from build123d import *

# Parameters (mm, degrees)
SKETCH1_W               = 129
SKETCH1_H               = 20
BOSS_EXTRUDE1_DEPTH     = 8
SKETCH2_W               = 13
SKETCH2_H               = 15
SKETCH2_W_2             = 12
SKETCH2_H_2             = 13
CUT_EXTRUDE4_DEPTH      = 3.6
SKETCH2_5_R             = 2.25
CUT_EXTRUDE7_DEPTH      = 131.786084887
CUT_EXTRUDE8_DEPTH      = 131.615313038
CUT_EXTRUDE8_DEPTH_BACK = 131.615313038
SKETCH3_W               = 13
SKETCH3_H               = 3
CUT_EXTRUDE9_DEPTH      = 5
CHAMFER1_SIZE           = 1
SKETCH5_W               = 42
SKETCH5_H               = 20
SKETCH5_W_2             = 2
SKETCH5_H_2             = 8
CUT_EXTRUDE10_DEPTH     = 2.5
CHAMFER2_DEPTH          = 20
SKETCH6_W               = 5
SKETCH6_H               = 4.5
SKETCH6_W_2             = 8
SKETCH6_H_2             = 3.5
CUT_EXTRUDE11_DEPTH     = 4
SKETCH7_W               = 20
SKETCH7_H               = 4
SKETCH7_W_2             = 10
SKETCH7_W_3             = 5
SKETCH7_H_2             = 5
BOSS_EXTRUDE2_DEPTH     = 2.5
CHAMFER3_SIZE           = 1
FILLET1_R               = 2
CHAMFER4_SIZE           = 1


with BuildPart() as part:
    # Sketch1 → Boss-Extrude1 (new body)
    with BuildSketch(Plane.XY):
        with Locations((64.5, 10)):
            Rectangle(SKETCH1_W, SKETCH1_H)
    extrude(amount=BOSS_EXTRUDE1_DEPTH)

    # Sketch2 → Cut-Extrude4 (cut)
    with BuildSketch(Plane.XY.offset(8)):
        with Locations((12.5, 8.5)):
            Rectangle(SKETCH2_W, SKETCH2_H)
        with Locations((55, 9.5)):
            Rectangle(SKETCH2_W_2, SKETCH2_H_2)
        with Locations((34, 9.5)):
            Rectangle(SKETCH2_W_2, SKETCH2_H_2)
        with Locations((76, 9.5)):
            Rectangle(SKETCH2_W_2, SKETCH2_H_2)
        with Locations((97, 9.5)):
            Rectangle(SKETCH2_W_2, SKETCH2_H_2)
        with BuildLine():
            Line((112, 16), (112, 3))
            Line((112, 3), (123.75, 3))
            ThreePointArc((123.75, 3), (123.813393039, 3.530330086), (124, 4.030776406))
            Line((124, 4.030776406), (124, 15.969223594))
            ThreePointArc((124, 15.969223594), (123.992158813, 15.984581975), (123.984435563, 16))
            Line((123.984435563, 16), (112, 16))
        make_face()
    extrude(amount=-CUT_EXTRUDE4_DEPTH, mode=Mode.SUBTRACT)

    # Sketch2<5> → Cut-Extrude7 (cut, through all)
    with BuildSketch(Plane.XY.offset(8)):
        with Locations((126, 3)):
            Circle(SKETCH2_5_R)
        with Locations((126, 17)):
            Circle(SKETCH2_5_R)
        with Locations((3, 17)):
            Circle(SKETCH2_5_R)
        with Locations((3, 3)):
            Circle(SKETCH2_5_R)
    extrude(amount=-CUT_EXTRUDE7_DEPTH, mode=Mode.SUBTRACT)

    # Sketch3 → Cut-Extrude8 (cut, two sides: drawn at the far end of the back side and taken through both)
    with BuildSketch(Plane.XY.offset(4.4).offset(-CUT_EXTRUDE8_DEPTH_BACK)):
        with Locations((12.5, 1.5)):
            Rectangle(SKETCH3_W, SKETCH3_H)
    extrude(amount=CUT_EXTRUDE8_DEPTH + CUT_EXTRUDE8_DEPTH_BACK, mode=Mode.SUBTRACT)

    # Sketch4 → Cut-Extrude9 (cut)
    with BuildSketch(Plane(origin=(0, 0, 0), x_dir=(-1, 0, 0), z_dir=(0, 0, -1))):
        with BuildLine():
            Line((-28.5, 4.596136616), (-28.5, 15.403863384))
            ThreePointArc((-28.5, 15.403863384), (-24.5, 19.403863384), (-20.5, 15.403863384))
            Line((-20.5, 15.403863384), (-20.5, 4.596136616))
            ThreePointArc((-20.5, 4.596136616), (-24.5, 0.596136616), (-28.5, 4.596136616))
        make_face()
    extrude(amount=-CUT_EXTRUDE9_DEPTH, mode=Mode.SUBTRACT)

    # Chamfer1
    # the kernel refuses this chamfer: 1 mm, written as the material it takes off along each edge
    with BuildSketch(Plane(origin=(24.5, 4.596136616, 0), x_dir=(-1, 0, 0), z_dir=(0, 1, 0))) as chamfer1_piece_1:
        Polygon((4 + CHAMFER1_SIZE, 0), (4, CHAMFER1_SIZE), (4, 0), align=None)
    revolve(axis=Axis((24.5, 4.596136616, 0), (0, 0, 1)), revolution_arc=180, mode=Mode.SUBTRACT)
    with BuildSketch(Plane(origin=(20.5, 15.403863384, 0), x_dir=(-1, 0, 0), z_dir=(0, -1, 0)), Plane(origin=(28.5, 4.596136616, 0), x_dir=(1, 0, 0), z_dir=(0, 1, 0))) as chamfer1_piece_2:
        Polygon((CHAMFER1_SIZE, 0), (0, -CHAMFER1_SIZE), (0, 0), align=None)
    extrude(amount=10.807726767, mode=Mode.SUBTRACT)
    with BuildSketch(Plane(origin=(24.5, 15.403863384, 0), x_dir=(1, 0, 0), z_dir=(0, -1, 0))) as chamfer1_piece_3:
        Polygon((4 + CHAMFER1_SIZE, 0), (4, CHAMFER1_SIZE), (4, 0), align=None)
    revolve(axis=Axis((24.5, 15.403863384, 0), (0, 0, 1)), revolution_arc=180, mode=Mode.SUBTRACT)

    # Sketch5 → Cut-Extrude10 (cut)
    with BuildSketch(Plane(origin=(0, 0, 0), x_dir=(-1, 0, 0), z_dir=(0, 0, -1))):
        with Locations((-49.5, 10)):
            Rectangle(SKETCH5_W, SKETCH5_H)
        with Locations((-1, 10)):
            Rectangle(SKETCH5_W_2, SKETCH5_H_2)
    extrude(amount=-CUT_EXTRUDE10_DEPTH, mode=Mode.SUBTRACT)

    # Chamfer2: read off the stored shape, not the designer's step
    # Chamfer2 outline → Chamfer2 (add)
    with BuildSketch(Plane(origin=(0, 0, 0), x_dir=(1, 0, 0), z_dir=(0, 1, 0))):
        Polygon((28.5, -1), (28.5, -2.5), (30, -2.5), align=None)
    extrude(amount=CHAMFER2_DEPTH)

    # Sketch6 → Cut-Extrude11 (cut)
    with BuildSketch(Plane(origin=(0, 0, 0), x_dir=(-1, 0, 0), z_dir=(0, 0, -1))):
        with Locations((-88.5, 4.75)):
            Rectangle(SKETCH6_W, SKETCH6_H)
        Polygon((-113, 2.5), (-108, 2.5), (-108, 12.5), (-113, 12.5), (-113, 10), (-113, 6), align=None)
        with Locations((-117, 4.25)):
            Rectangle(SKETCH6_W_2, SKETCH6_H_2)
        Polygon((-121, 6), (-113, 6), (-113, 10), (-129, 10), (-129, 6), align=None)
        Polygon((-113, 10), (-113, 12.5), (-113, 14), (-129, 14), (-129, 10), align=None)
    extrude(amount=-CUT_EXTRUDE11_DEPTH, mode=Mode.SUBTRACT)

    # Sketch7 → Boss-Extrude2 (add)
    with BuildSketch(Plane(origin=(0, 0, 2.5), x_dir=(-1, 0, 0), z_dir=(0, 0, -1))):
        with Locations((-60.5, 2)):
            Rectangle(SKETCH7_W, SKETCH7_H)
        with Locations((-65.5, 18)):
            Rectangle(SKETCH7_W_2, SKETCH7_H)
        with Locations((-43.5, 8.5)):
            Rectangle(SKETCH7_W_3, SKETCH7_H_2)
    extrude(amount=BOSS_EXTRUDE2_DEPTH)

    # Chamfer3
    chamfer3_edges = [part.edges().sort_by_distance(p)[0] for p in [
        (0, 14, 1.25),
        (0, 6, 1.25),
    ]]
    chamfer(chamfer3_edges, length=CHAMFER3_SIZE)

    # Fillet1
    fillet1_edges = [part.edges().sort_by_distance(p)[0] for p in [
        (112, 3, 6.2),
        (112, 16, 6.2),
        (70, 16, 6.2),
        (82, 16, 6.2),
        (82, 3, 6.2),
        (70, 3, 6.2),
        (40, 16, 6.2),
        (40, 3, 6.2),
        (61, 16, 6.2),
        (61, 3, 6.2),
        (49, 3, 6.2),
        (49, 16, 6.2),
        (103, 16, 6.2),
        (103, 3, 6.2),
        (91, 3, 6.2),
        (91, 16, 6.2),
    ]]
    fillet(fillet1_edges, radius=FILLET1_R)

    # Chamfer4
    chamfer4_edges = [part.edges().sort_by_distance(p)[0] for p in [
        (0, 20, 4),
        (129, 20, 4),
        (129, 0, 4),
        (0, 0, 4),
    ]]
    chamfer(chamfer4_edges, length=CHAMFER4_SIZE)


solid = part.part
Input: part model. Units: mm. Frame: model coordinates. A direction names the side the tool comes from. Coordinates: 2 decimals unless noted, no trailing zeros. Order: outer loops, then holes, each group sorted by start corner. A loop starts at its lowest first (then second) coordinate and runs counter-clockwise, first axis right, second up. Notation, with made-up numbers: M 82.5,52.5 L 134.5,52.5 A24 ccw 134.5,75.5 Z; hole C 24,-33 d6. An arc over 180 degrees is marked long. Answer as CSV lines item,"result".
1. Material intervals for line 1 (Y direction, x = 3, z = 5.5); line 2 (Y direction, x = 126, z = 3.25); line 3 (X direction, y = 6.5, z = 1.25), sorted ascending. Write a range as from..to.
Reported:
line 1,"0..0.75, 5.25..14.75, 19.25..20"
line 2,"0..0.75, 5.25..6, 14..14.75, 19.25..20"
line 3,"2..20.5, 28.5..28.75, 41..46, 70.5..86, 91..108"
2. Section B-B (x = 74.5). Return the cut outline in (y, z), then the cut area to 3 significant figures.
Reported:
outline,"M 0,0 L 20,0 L 20,8 L 16,8 L 16,4.4 L 3,4.4 L 3,8 L 0,8 Z"
area,"113 mm2"
3. Section D-D (x = 24.5). Return the cut outline in (y, z).
Reported:
outline,"M 0,0.4 L 0.6,1 L 0.6,5 L 19.4,5 L 19.4,1 L 20,0.4 L 20,8 L 0,8 Z"
4. Access query for faces 1 (the flat face through (76, 3, 6)), 2 (the flat face through (12, 10, 4.4)), 3 (the flat face through (46, 8, 1)), 4 (the flat face through (1, 10, 2.5)). Directions: +Z, -Z, +X, -X, +Y, -Y. A direction counts if a zero-diameter tool reaches every point of the face in a straight line with its end or side. Return the directions, or none.
Reported:
face 1,"+Z"
face 2,"+Z, -Y"
face 3,"-Z, +Y, -Y"
face 4,"-Z, -X"
5. Section A-A (x = 126). Return the cut outline in (y, z).
Reported:
outline,"M 0,0 L 0.75,0 L 0.75,8 L 0,8 Z; M 5.25,0 L 6,0 L 6,4 L 14,4 L 14,0 L 14.75,0 L 14.75,8 L 5.25,8 Z; M 19.25,0 L 20,0 L 20,8 L 19.25,8 Z"
6. First-contact query: P1, Ø1.8, axis at x = 12, z = 7, coming from the -Y side; P2, Ø3.5, axis at x = 14.5, z = 2.5, coming from the -Y side; P3, Ø1.3, axis at x = 88.5, y = 4.5, coming from the -Z side. Flat tips, straight axial feed; report the tip coordinate or a pass-through.
Reported:
P1,"y = 16"
P2,"y = 3"
P3,"z = 4"
7. Section C-C (z = 6.25). State how many separate pieces and enclosed holes the cut face has, then the cut area to 3 significant figures.
Reported:
separate pieces,"1"
enclosed holes,"7"
area,"1,540 mm2"
8. Pull-direction query (Y, two-part tool) for faces 5 (the flat face through (6, 6, 6)), 6 (the flat face through (74, 0, 4)), 7 (the cylindrical face through (91.6, 15.43, 6.17)), 8 (the flat face through (2, 10, 1)); classes: released by +Y, released by -Y, zero draft, split by the parting line, or undercut.
Reported:
face 5,"zero draft"
face 6,"released by -Y"
face 7,"undercut"
face 8,"undercut"
